from build123d import *

# Parameters (mm, degrees)
SKETCH1_W                      = 60
SKETCH1_H                      = 335.5
BASE_FLANGE1_DEPTH             = 3
EDGE_FLANGE1_STRIP_W           = 14
EDGE_FLANGE1_STRIP_H           = 3
EDGE_FLANGE1_STRIP_CUT_DEPTH   = 335.5
EDGE_FLANGE1_DEPTH             = 335.5
EDGE_FLANGE2_STRIP_W           = 14
EDGE_FLANGE2_STRIP_H           = 3
EDGE_FLANGE2_STRIP_CUT_DEPTH   = 56
EDGE_FLANGE2_STRIP_2_W         = 14
EDGE_FLANGE2_STRIP_2_H         = 3
EDGE_FLANGE2_STRIP_CUT_2_DEPTH = 56
EDGE_FLANGE2_STRIP_3_W         = 14
EDGE_FLANGE2_STRIP_3_H         = 3
EDGE_FLANGE2_STRIP_CUT_3_DEPTH = 56
EDGE_FLANGE2_STRIP_4_W         = 14
EDGE_FLANGE2_STRIP_4_H         = 3
EDGE_FLANGE2_STRIP_CUT_4_DEPTH = 56
EDGE_FLANGE2_DEPTH             = 56
EDGE_FLANGE2_BEND_DEPTH        = 56
EDGE_FLANGE2_BEND_2_DEPTH      = 56
EDGE_FLANGE2_BEND_3_DEPTH      = 56
SKETCH18_R                     = 4.6
EXTRUDE1_DEPTH                 = 348.346009046
SKETCH21_R                     = 4.6
CUT_EXTRUDE1_DEPTH             = 10
SKETCH22_R                     = 4.6
CUT_EXTRUDE2_DEPTH             = 10


# Sheet-metal steps are written as plain solids
with BuildPart() as part:
    # Sketch1 → Base-Flange1 (new body)
    with BuildSketch(Plane(origin=(0, 0, 0), x_dir=(1, 0, 0), z_dir=(0, 1, 0))):
        Rectangle(SKETCH1_W, SKETCH1_H)
    extrude(amount=BASE_FLANGE1_DEPTH)

    # Edge-Flange1 strip (across the edge) → Edge-Flange1 strip cut (cut)
    with BuildSketch(Plane(origin=(-30, 3, -167.75), x_dir=(1, 0, 0), z_dir=(0, 0, 1))):
        with Locations((-3, -1.5)):
            Rectangle(EDGE_FLANGE1_STRIP_W, EDGE_FLANGE1_STRIP_H)
    extrude(amount=EDGE_FLANGE1_STRIP_CUT_DEPTH, mode=Mode.SUBTRACT)

    # Edge-Flange1 section (across the edge) → Edge-Flange1 (add)
    with BuildSketch(Plane(origin=(-30, 3, -167.75), x_dir=(1, 0, 0), z_dir=(0, 0, 1))):
        with BuildLine():
            Line((0, 1), (0, 57))
            Line((0, 57), (3, 57))
            Line((3, 57), (3, 1))
            ThreePointArc((3, 1), (3.292893219, 0.292893219), (4, 0))
            Line((4, 0), (4, -3))
            ThreePointArc((4, -3), (1.171572875, -1.828427125), (0, 1))
        make_face()
    extrude(amount=EDGE_FLANGE1_DEPTH)

    # Edge-Flange2 strip (across the edge) → Edge-Flange2 strip cut (cut)
    with BuildSketch(Plane(origin=(-30, 4, 167.75), x_dir=(0, 0, -1), z_dir=(0, 1, 0))):
        with Locations((-3, -1.5)):
            Rectangle(EDGE_FLANGE2_STRIP_W, EDGE_FLANGE2_STRIP_H)
    extrude(amount=EDGE_FLANGE2_STRIP_CUT_DEPTH, mode=Mode.SUBTRACT)

    # Edge-Flange2 strip 2 (across the edge) → Edge-Flange2 strip cut 2 (cut)
    with BuildSketch(Plane(origin=(30, 0, 167.75), x_dir=(0, 0, -1), z_dir=(-1, 0, 0))):
        with Locations((-3, -1.5)):
            Rectangle(EDGE_FLANGE2_STRIP_2_W, EDGE_FLANGE2_STRIP_2_H)
    extrude(amount=EDGE_FLANGE2_STRIP_CUT_2_DEPTH, mode=Mode.SUBTRACT)

    # Edge-Flange2 strip 3 (across the edge) → Edge-Flange2 strip cut 3 (cut)
    with BuildSketch(Plane(origin=(-30, 60, -167.75), x_dir=(0, 0, 1), z_dir=(0, -1, 0))):
        with Locations((-3, -1.5)):
            Rectangle(EDGE_FLANGE2_STRIP_3_W, EDGE_FLANGE2_STRIP_3_H)
    extrude(amount=EDGE_FLANGE2_STRIP_CUT_3_DEPTH, mode=Mode.SUBTRACT)

    # Edge-Flange2 strip 4 (across the edge) → Edge-Flange2 strip cut 4 (cut)
    with BuildSketch(Plane(origin=(-26, 0, -167.75), x_dir=(0, 0, 1), z_dir=(1, 0, 0))):
        with Locations((-3, -1.5)):
            Rectangle(EDGE_FLANGE2_STRIP_4_W, EDGE_FLANGE2_STRIP_4_H)
    extrude(amount=EDGE_FLANGE2_STRIP_CUT_4_DEPTH, mode=Mode.SUBTRACT)

    # Edge-Flange2 section (across the edge) → Edge-Flange2 (add)
    with BuildSketch(Plane(origin=(-30, 4, 167.75), x_dir=(0, 0, -1), z_dir=(0, 1, 0))):
        with BuildLine():
            Line((0, 1), (0, 37))
            Line((0, 37), (3, 37))
            Line((3, 37), (3, 1))
            ThreePointArc((3, 1), (3.292893219, 0.292893219), (4, 0))
            Line((4, 0), (4, -3))
            ThreePointArc((4, -3), (1.171572875, -1.828427125), (0, 1))
        make_face()
    extrude(amount=EDGE_FLANGE2_DEPTH)

    # Edge-Flange2 section 2 (across the edge) → Edge-Flange2 bend (add)
    with BuildSketch(Plane(origin=(30, 0, 167.75), x_dir=(0, 0, -1), z_dir=(-1, 0, 0))):
        with BuildLine():
            Line((0, 1), (0, 37))
            Line((0, 37), (3, 37))
            Line((3, 37), (3, 1))
            ThreePointArc((3, 1), (3.292893219, 0.292893219), (4, 0))
            Line((4, 0), (4, -3))
            ThreePointArc((4, -3), (1.171572875, -1.828427125), (0, 1))
        make_face()
    extrude(amount=EDGE_FLANGE2_BEND_DEPTH)

    # Edge-Flange2 section 3 (across the edge) → Edge-Flange2 bend 2 (add)
    with BuildSketch(Plane(origin=(-30, 60, -167.75), x_dir=(0, 0, 1), z_dir=(0, -1, 0))):
        with BuildLine():
            Line((0, 1), (0, 37))
            Line((0, 37), (3, 37))
            Line((3, 37), (3, 1))
            ThreePointArc((3, 1), (3.292893219, 0.292893219), (4, 0))
            Line((4, 0), (4, -3))
            ThreePointArc((4, -3), (1.171572875, -1.828427125), (0, 1))
        make_face()
    extrude(amount=EDGE_FLANGE2_BEND_2_DEPTH)

    # Edge-Flange2 section 4 (across the edge) → Edge-Flange2 bend 3 (add)
    with BuildSketch(Plane(origin=(-26, 0, -167.75), x_dir=(0, 0, 1), z_dir=(1, 0, 0))):
        with BuildLine():
            Line((0, 1), (0, 37))
            Line((0, 37), (3, 37))
            Line((3, 37), (3, 1))
            ThreePointArc((3, 1), (3.292893219, 0.292893219), (4, 0))
            Line((4, 0), (4, -3))
            ThreePointArc((4, -3), (1.171572875, -1.828427125), (0, 1))
        make_face()
    extrude(amount=EDGE_FLANGE2_BEND_3_DEPTH)

    # Sketch18 → Extrude1 (cut, through all)
    with BuildSketch(Plane.XY.offset(167.75)):
        with Locations((-47, 47.5)):
            Circle(SKETCH18_R)
        with Locations((-47, 17.5)):
            Circle(SKETCH18_R)
        with Locations((-12.5, -17)):
            Circle(SKETCH18_R)
        with Locations((17.5, -17)):
            Circle(SKETCH18_R)
    extrude(amount=-EXTRUDE1_DEPTH, mode=Mode.SUBTRACT)

    # Sketch21 → Cut-Extrude1 (cut)
    with BuildSketch(Plane.XZ):
        with Locations(Location((5, -87.75, 0), (0, 0, 270))):
            Circle(SKETCH21_R)
        with Locations(Location((5, 117.75, 0), (0, 0, 270))):
            Circle(SKETCH21_R)
    extrude(amount=-CUT_EXTRUDE1_DEPTH, mode=Mode.SUBTRACT)

    # Sketch22 → Cut-Extrude2 (cut)
    with BuildSketch(Plane.ZY.offset(30)):
        with Locations(Location((-87.75, 35, 0), (0, 0, 270))):
            Circle(SKETCH22_R)
        with Locations(Location((117.75, 35, 0), (0, 0, 270))):
            Circle(SKETCH22_R)
    extrude(amount=-CUT_EXTRUDE2_DEPTH, mode=Mode.SUBTRACT)


solid = part.part
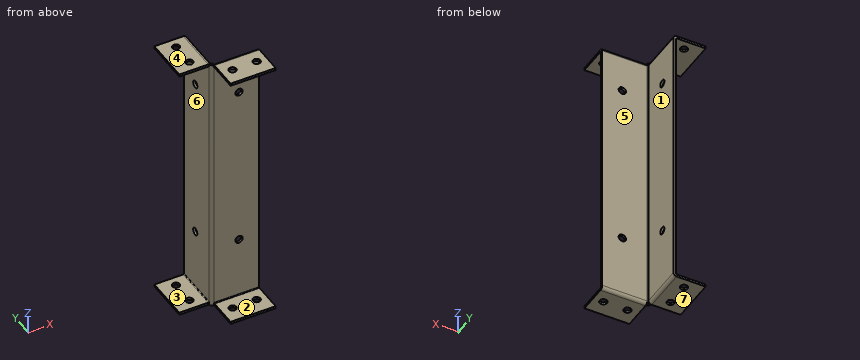
The listing builds one solid part. Answer for the finished solid, in the listing's coordinates (mm). Face numbers are marked on the shaded views. A direction names the side the tool comes from. Give positions to 0.01 mm unless a question says otherwise; leave off trailing zeros. Write each loop counter-clockwise with the first axis right and the second up, starting at its lowest first coordinate (ties: lowest second). Pieces come first, ordered by that corner, then holes.
1) For a pull along Z with two mould halves and no side action, classify the marked faces 4, 5, 6 and 7 as pulls with the +Z half, pulls with the -Z half, needs draft (parallel to the pull), parting line crosses it, or undercut.
2) Find the intervals of material crossed by L1, parallel to Y at x = -47, z = -166.4; L2, parallel to Z at x = 5, y = -28; L3, parallel to Y at x = 15, z = 75, in increasing order.
3) Given P1, Ø5, axis at x = -8, z = 92.5, coming from the -Y side; P2, Ø3, axis at x = -54.5, z = -166, coming from the -Y side; P3, Ø7.5, axis at y = 35, z = -87.75, coming from the +X side; P4, Ø2, axis at y = -21, z = -165, coming from the -X side, each flat-ended and moving along its own axis, determine where each tip first touches the part or whether it passes through.
4) Section D-D (x = 5) is taken. Write down the section's boundary in (y, z), and give its area (3 significant figures).
5) Section A-A (x = -47) is taken. Write down the section's boundary in (y, z).
6) Section C-C (y = -17) is taken. Write down the section's boundary in (x, z).
7) A tool of negligible diameter and unlimited length cuts with its end or side. For the marked faces 1, 2 and 3, from which of +Z, -Z, +X, -X, +Y, -Y can it reach the whole face along a straight path? Write none if from no direction.
8) Section B-B (z = -87.75) is taken. Write down the section's boundary in (x, y), and give its area (3 significant figures).
Response:
1. face 4: pulls with the +Z half
1. face 5: needs draft
1. face 6: undercut
1. face 7: pulls with the -Z half
2. L1: y = 4 to 12.9, 22.1 to 42.9, 52.1 to 60
2. L2: z = -167.75 to -164.75, 164.75 to 167.75
2. L3: y = 0 to 3
3. P1: stops at y = 0
3. P2: stops at y = 4
3. P3: passes through
3. P4: stops at x = -26
4. outline: (-37, -167.75) - (-1, -167.75) arc R4 ccw to (3, -163.75) - (3, -92.35) - (0, -92.35) - (0, -163.75) arc R1 cw to (-1, -164.75) - (-37, -164.75) - close; (-37, 164.75) - (-1, 164.75) arc R1 cw to (0, 163.75) - (0, 122.35) - (3, 122.35) - (3, 163.75) arc R4 ccw to (-1, 167.75) - (-37, 167.75) - close; (0, -83.15) - (3, -83.15) - (3, 113.15) - (0, 113.15) - close
4. area: 1,170 mm2
5. outline: (4, -167.75) - (12.9, -167.75) - (12.9, -164.75) - (4, -164.75) - close; (4, 164.75) - (12.9, 164.75) - (12.9, 167.75) - (4, 167.75) - close; (22.1, -167.75) - (42.9, -167.75) - (42.9, -164.75) - (22.1, -164.75) - close; (22.1, 164.75) - (42.9, 164.75) - (42.9, 167.75) - (22.1, 167.75) - close; (52.1, -167.75) - (60, -167.75) - (60, -164.75) - (52.1, -164.75) - close; (52.1, 164.75) - (60, 164.75) - (60, 167.75) - (52.1, 167.75) - close
6. outline: (-26, -167.75) - (-17.1, -167.75) - (-17.1, -164.75) - (-26, -164.75) - close; (-26, 164.75) - (-17.1, 164.75) - (-17.1, 167.75) - (-26, 167.75) - close; (-7.9, -167.75) - (12.9, -167.75) - (12.9, -164.75) - (-7.9, -164.75) - close; (-7.9, 164.75) - (12.9, 164.75) - (12.9, 167.75) - (-7.9, 167.75) - close; (22.1, -167.75) - (30, -167.75) - (30, -164.75) - (22.1, -164.75) - close; (22.1, 164.75) - (30, 164.75) - (30, 167.75) - (22.1, 167.75) - close
7. face 1: +Z, -Z, +X, +Y
7. face 2: +X, -X, -Y
7. face 3: -X, +Y, -Y
8. outline: (-30, 4) arc R4 ccw to (-26, 0) - (0.4, 0) - (0.4, 3) - (-26, 3) arc R1 cw to (-27, 4) - (-27, 30.4) - (-30, 30.4) - close; (-30, 39.6) - (-27, 39.6) - (-27, 60) - (-30, 60) - close; (9.6, 0) - (30, 0) - (30, 3) - (9.6, 3) - close
8. area: 293 mm2
